from build123d import *

# Parameters (mm, degrees)
SKETCH_W        = 10.8
SKETCH_H        = 10.8
PAD_DEPTH       = 10.8
THICKNESS_T     = 1
SKETCH001_W     = 10.8
SKETCH001_H     = 1
PAD001_DEPTH    = 6
SKETCH002_R     = 1.4
POCKET_DEPTH    = 1.001
SKETCH003_W     = 10.8
SKETCH003_H     = 3.3
POCKET001_DEPTH = 1.001
SKETCH004_W     = 4.8
SKETCH004_H     = 4.8
POCKET002_DEPTH = 1
SKETCH005_W     = 4.8
SKETCH005_H     = 4.8
POCKET003_DEPTH = 12.801


with BuildPart() as part:
    # Sketch → Pad (new body)
    with BuildSketch(Plane.XY):
        with Locations((5.4, 5.4)):
            Rectangle(SKETCH_W, SKETCH_H)
    extrude(amount=PAD_DEPTH)

    # Thickness
    thickness_openings = [part.faces().sort_by_distance(p)[0] for p in [
        (5.4, 5.4, 10.8),
    ]]
    offset(amount=THICKNESS_T, openings=thickness_openings)

    # Sketch001 → Pad001 (new body)
    with BuildSketch(Plane.XY.offset(10.8)):
        with Locations((5.4, 11.3)):
            Rectangle(SKETCH001_W, SKETCH001_H)
    extrude(amount=PAD001_DEPTH)

    # Sketch002 → Pocket (cut, through all)
    with BuildSketch(Plane.XZ.offset(-10.8)):
        with Locations((5.4, 13.8)):
            Circle(SKETCH002_R)
    extrude(amount=-POCKET_DEPTH, mode=Mode.SUBTRACT)

    # Sketch003 → Pocket001 (cut, through all)
    with BuildSketch(Plane.XY):
        with Locations((5.4, 9.15)):
            Rectangle(SKETCH003_W, SKETCH003_H)
    extrude(amount=-POCKET001_DEPTH, mode=Mode.SUBTRACT)

    # Sketch004 → Pocket002 (cut)
    with BuildSketch(Plane.XZ.offset(1)):
        with Locations((5.4, 5.4)):
            Rectangle(SKETCH004_W, SKETCH004_H)
    extrude(amount=-POCKET002_DEPTH, mode=Mode.SUBTRACT)

    # Sketch005 → Pocket003 (cut, through all)
    with BuildSketch(Plane.YZ.offset(11.8)):
        with Locations((5.4, 5.4)):
            Rectangle(SKETCH005_W, SKETCH005_H)
    extrude(amount=-POCKET003_DEPTH, mode=Mode.SUBTRACT)


solid = part.part
The model under review builds one solid part; all positions refer to its coordinate system, in mm. A direction names the side the tool comes from. Coordinates: 2 decimals unless noted, no trailing zeros. Write each loop counter-clockwise with the first axis right and the second up, starting at its lowest first coordinate (ties: lowest second). Pieces come first, ordered by that corner, then holes. Notation, with made-up numbers: (20, 16.25) - (73, 16.25) arc R24 ccw to (73, 43.25) - close; hole circle Ø2 at (-12, -35.75). An arc over 180 degrees is marked (long way). Answer as a JSON object with one key per item and string values. Group by question number.
1. Add section D-D (z = 13.8). Give the boundary of the cut face in (x, y).
2. Clearance check with flat-ended pins moving along their axes: pin 1 Ø0.5 at (x, y) = (-0.5, 4.5) entering from +Z; pin 2 Ø2 at (x, y) = (3, 5.5) entering from +Z; pin 3 Ø1.1 at (y, z) = (11, 13) entering from +X. State where each tip first meets the part, or that it passes through.
3. Add section B-B (x = 5.4). Give the boundary of the cut face in (y, z).
4. To check wall thickness, follow probe 1 along X at (y, z) = (4.75, 8.75); probe 2 along Y at (x, z) = (1.5, 11.5). State the ranges of each line that lie inside material, in increasing order.
5. Machinability: for faces 1 (the face through (-0.5, 7.8, 5.4)), 2 (the face through (5, 4, 0)), 3 (the face through (5.4, -0.5, 3)), 4 (the face through (-0.715, 11.499, 5.476)), 5 (the face through (5, 4, -1)), which of the approach directions +Z, -Z, +X, -X, +Y, -Y give a long, thin tool a straight path to every point of the face, cutting with its end or side? Answer none if there is none.
6. Mouldability with a two-part tool opening along X and no side actions: class faces 6 (the face through (-0.715, -0.699, 5.476)), 7 (the face through (5, 11.8, 8)), 8 (the face through (0, 5, 2)), 9 (the face through (5, 10.8, 8)) as pulls with the +X half, pulls with the -X half, needs draft (parallel to the pull), parting line crosses it, or undercut.
7. Add section C-C (z = 5). Give the boundary of the cut face in (x, y).
8. Add section A-A (y = 9.75). Give the boundary of the cut face in (x, z), plus the area to 3 significant figures.
Findings:
{
 "1": {"outline": "(0, 10.8) - (4, 10.8) - (4, 11.8) - (0, 11.8) - close; (6.8, 10.8) - (10.8, 10.8) - (10.8, 11.8) - (6.8, 11.8) - close"},
 "2": {"pin 1": "z = 10.8", "pin 2": "z = 0", "pin 3": "x = 10.8"},
 "3": {"outline": "(-1, 0) arc R1 ccw to (0, -1) - (7.5, -1) - (7.5, 0) - (0, 0) - (0, 3) - (-1, 3) - close; (-1, 7.8) - (0, 7.8) - (0, 10.8) - (-1, 10.8) - close; (10.8, -1) arc R1 ccw to (11.8, 0) - (11.8, 12.4) - (10.8, 12.4) - close; (10.8, 15.2) - (11.8, 15.2) - (11.8, 16.8) - (10.8, 16.8) - close"},
 "4": {"probe 1": "-1 to 0, 10.8 to 11.8", "probe 2": "10.8 to 11.8"},
 "5": {"face 1": "+X, -X", "face 2": "+Z", "face 3": "-Y", "face 4": "+Z, -Z, -X, +Y", "face 5": "-Z, +X, -X, +Y, -Y"},
 "6": {"face 6": "pulls with the -X half", "face 7": "needs draft", "face 8": "undercut", "face 9": "undercut"},
 "7": {"outline": "(-1, 0) arc R1 ccw to (0, -1) - (3, -1) - (3, 0) - (0, 0) - (0, 3) - (-1, 3) - close; (-1, 7.8) - (0, 7.8) - (0, 10.8) - (10.8, 10.8) - (10.8, 7.8) - (11.8, 7.8) - (11.8, 10.8) arc R1 ccw to (10.8, 11.8) - (0, 11.8) arc R1 ccw to (-1, 10.8) - close; (7.8, -1) - (10.8, -1) arc R1 ccw to (11.8, 0) - (11.8, 3) - (10.8, 3) - (10.8, 0) - (7.8, 0) - close"},
 "8": {"outline": "(-1, 0) arc R1 ccw to (0, -1) - (0, 10.8) - (-1, 10.8) - close; (10.8, -1) arc R1 ccw to (11.8, 0) - (11.8, 10.8) - (10.8, 10.8) - close", "area": "23.2 mm²"}
}
